Input: part model. Units: mm. Frame: model coordinates. A direction names the side the tool comes from. Coordinates: 2 decimals unless noted, no trailing zeros. Write each loop counter-clockwise with the first axis right and the second up, starting at its lowest first coordinate (ties: lowest second). Pieces come first, ordered by that corner, then holes. Notation, with made-up numbers: (-5, 21.5) - (42, 21.5) arc R26 ccw to (42, 35.5) - close; hole circle Ø9 at (-16, 84). An arc over 180 degrees is marked (long way). Use a Markdown table: item, result. Add a question column.
Q1. Section query A-A (z = 31.5). Return the cut outline in (x, y) (3 decimals).
Q2. Set-up query: faces 1 (the face through (11.28, 26.65, 42.43)), 2 (the face through (0.29, 4.52, 42.01)), 3 (the face through (1, 0.635, 42)). Return all of +Z, -Z, +X, -X, +Y, -Y with unobstructed straight access to the full face (end or side cutting, diameter ignored); none if empty.
Q3. Mould query, pull axis Y, two halves, no side actions, for faces 4 (the face through (-2, 0.635, 30)), 5 (the face through (-11.953, 26.012, 30.239)), 6 (the face through (-6, 38.735, 34)). Classes: released by +Y, released by -Y, zero draft, split by the parting line, or undercut.
Q4. Section query C-C (y = 12). Return the cut outline in (x, z), then the cut area to 3 significant figures.
Q5. Section query D-D (y = 27). Return the cut outline in (x, z).
Q6. Pin query (flat end, axial travel): P1, Ø10, axis at x = -7, y = 29, coming from the -Z side; P2, Ø9, axis at x = 6.29, z = 42.21, coming from the -Y side; P3, Ø4, axis at y = -8, z = 20, coming from the +X side. Return the tip coordinate at first contact, or that it passes through.
Q7. Material intervals for probe 1 along X at (y, z) = (4, 43.5); probe 2 along X at (y, z) = (21, 42); probe 3 along Y at (x, z) = (0, 52.5) (3 decimals), sorted ascending. Write a range as from..to.
Q8. Section query B-B (x = 4.75). Return the cut outline in (y, z) (3 decimals).
Autodesk Inventor part; units mm, degrees
ref_plane "Start Plane" through (0, 0, 0) normal (0, 0, 1) x (1, 0, 0)
ref_plane "End Plane" through (0, 0, 70.7107) normal (0, 0, 1) x (1, 0, 0)
ref_plane "Work Plane4" through (0, 13.335, 0) normal (0, 1, 0) x (-1, 0, 0)
ref_plane "Start Plane" through (0, 0, 0) normal (0, 0, 1) x (1, 0, 0)
ref_plane "End Plane" through (0, 0, 70.7107) normal (0, 0, 1) x (1, 0, 0)
sketch "Sketch" plane through (0, 0, 0) normal (0, 0, 1) x (1, 0, 0)
  circle A0 centre (0, 0) radius 10.4648
  circle A1 centre (0, 0) radius 13.335
  dimension "d0" = 26.67
  dimension "d1" = 2.8702
extrude "Body" add sketch "Sketch" along normal up to surface (70.7107 mm away) from surface at 0
sketch "Sketch3" plane through (0, 0, 0) normal (0, 0, 1) x (1, 0, 0)
  line L0 (0, 0) -> (10, 0)
ref_plane "Work Plane3" through (0, 0, 0) normal (0, -1, 0) x (1, 0, 0)
ref_plane "Work Plane4" through (0, 13.335, 0) normal (0, 1, 0) x (-1, 0, 0)
sketch "Sketch7" plane through (0, 13.335, 0) normal (0, 1, 0) x (-1, 0, 0)
  line L0 (-20.6433, 0) -> (18.9981, 0) construction
  line L1 (0, -14.1421) -> (0, 84.8528) construction
  line L2 (0, 0) -> (17.9605, 17.9605)
  line L3 (17.9605, 17.9605) -> (7.1842, 28.7368) construction
  circle A0 centre (7.1842, 28.7368) radius 5
  line L4 (7.1842, 28.7368) -> (-6.2862, 42.2072) construction
  circle A1 centre (7.1842, 28.7368) radius 6
  circle A2 centre (-6.2862, 42.2072) radius 5
  circle A3 centre (-6.2862, 42.2072) radius 6
  dimension "d23" = 45
  dimension "d24" = 25.4
  dimension "d25" = 15.24
  dimension "d26" = 19.05
  dimension "d28" = 12
  dimension "d29" = 10
extrude "Extrusion3" add sketch "Sketch7" along normal blind 25.4 and the other way blind 12.7
sketch "Sketch4" plane through (0, 0, 0) normal (0, -1, 0) x (1, 0, 0)
  line L0 (-2, 0) -> (12, 0)
  line L1 (-2, 70.7107) -> (12, 70.7107)
  dimension "d7" = 70.7107
equation "\"d0\" = G_H"
equation "\"d1\" = G_T"
equation "\"d2\" = G_L"
equation "\"G_H\" = 26.67"
equation "\"G_T\" = 2.8702"
equation "\"G_L\" = d7"
equation "\"G_OFFSET_START\" = 0"
equation "\"G_OFFSET_END\" = 0"
equation "\"d5\" = G_OFFSET_END + B_L"
equation "\"B_L\" = 70.71068"
properties part number "ANSI - 3/4 x 0.113 - 2.784" material "Steel, Mild"
Values follow:
| question | item | result |
|---|---|---|
| 1 | outline | (-12.51, 4.617) arc R13.335 ccw (long way) to (-1.858, 13.205) - (-1.858, 38.735) - (-3.017, 38.735) - (-3.017, 12.989) arc R13.335 ccw to (-11.351, 6.998) - (-11.351, 38.735) - (-12.51, 38.735) - close; hole (-3.017, 0.635) - (-3.017, 10.02) arc R10.465 ccw (long way) to (-1.858, 10.298) - (-1.858, 0.635) - close |
| 2 | face 1 | +Y |
| 2 | face 2 | none |
| 2 | face 3 | +Z, -Z |
| 3 | face 4 | undercut |
| 3 | face 5 | zero draft |
| 3 | face 6 | released by +Y |
| 4 | outline | (-5.82, 0) - (5.82, 0) - (5.82, 36.23) arc R6 ccw (long way) to (5.82, 48.19) - (5.82, 70.71) - (-5.82, 70.71) - (-5.82, 34.58) arc R6 ccw (long way) to (-5.82, 22.89) - close; hole (-5.82, 23.93) - (-5.82, 33.55) arc R5 ccw (long way) to start; hole (5.82, 37.23) arc R5 ccw (long way) to (5.82, 47.19) - close |
| 4 | area | 861 mm2 |
| 5 | outline | circle Ø12 at (-7.18, 28.74); circle Ø12 at (6.29, 42.21); hole circle Ø10 at (-7.18, 28.74); hole circle Ø10 at (6.29, 42.21) |
| 6 | P1 | z = 22.74 |
| 6 | P2 | y = -13.21 |
| 6 | P3 | x = 11.91 |
| 7 | probe 1 | -12.72..-9.67, 0.43..1.46, 9.67..12.72 |
| 7 | probe 2 | 0.29..1.29, 11.28..12.28 |
| 7 | probe 3 | -13.335..-10.465, 10.465..13.335 |
| 8 | outline | (-12.46, 0) - (-9.325, 0) - (-9.325, 70.711) - (-12.46, 70.711) - close; (0.635, 36.407) - (9.325, 36.407) - (9.325, 0) - (12.46, 0) - (12.46, 36.407) - (38.735, 36.407) - (38.735, 37.449) - (12.46, 37.449) - (12.46, 46.965) - (38.735, 46.965) - (38.735, 48.007) - (12.46, 48.007) - (12.46, 70.711) - (9.325, 70.711) - (9.325, 48.007) - (0.635, 48.007) - (0.635, 46.965) - (9.325, 46.965) - (9.325, 37.449) - (0.635, 37.449) - close |
